Design review of the part shown in the three views and the two pictorial views. Dimensions are in mm from the part's minimum x, y and z. Give positions to 0.01 mm unless a question says otherwise; leave off trailing zeros. Order: outer loops, then holes, each group sorted by start corner. A loop starts at its lowest first (then second) coordinate and runs counter-clockwise, first axis right, second up.
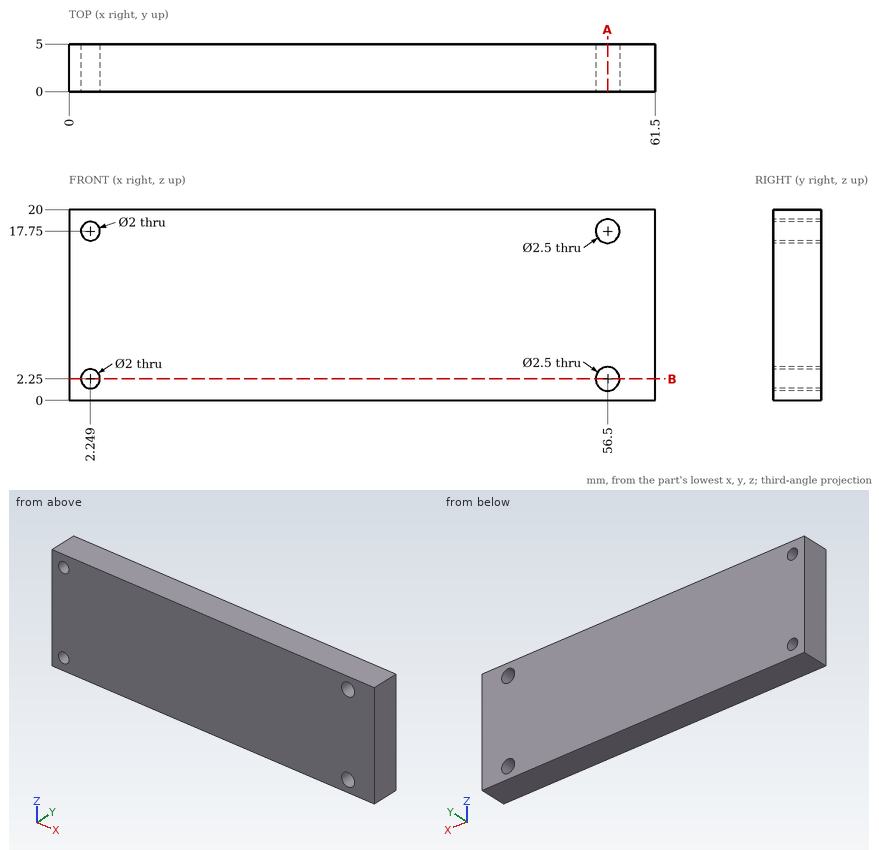
Item 1: Take a section at A-A (x = 56.5). Give the boundary of the cut face in (y, z), and give its area (3 significant figures).
Values found:
outline: (0, 0) - (5, 0) - (5, 1) - (0, 1) - close; (0, 3.5) - (5, 3.5) - (5, 16.5) - (0, 16.5) - close; (0, 19) - (5, 19) - (5, 20) - (0, 20) - close
area: 75.0 mm2
Item 2: Take a section at B-B (z = 2.25). Give the boundary of the cut face in (x, y).
Values found:
outline: (0, 0) - (1.25, 0) - (1.25, 5) - (0, 5) - close; (3.25, 0) - (55.25, 0) - (55.25, 5) - (3.25, 5) - close; (57.75, 0) - (61.5, 0) - (61.5, 5) - (57.75, 5) - close
Item 3: For line 1 (Z direction, x = 56.5, y = 1.25); line 2 (X direction, y = 3.15, z = 17.75); line 3 (X direction, y = 1.65, z = 18.5), list the stretches that pass through material, from the lowest coordinate up.
Values found:
line 1: z = 0 to 1, 3.5 to 16.5, 19 to 20
line 2: x = 0 to 1.25, 3.25 to 55.25, 57.75 to 61.5
line 3: x = 0 to 1.59, 2.91 to 55.5, 57.5 to 61.5
Item 4: Clearance check with flat-ended pins moving along their axes: pin 1 Ø3 at (x, z) = (56.5, 2.25) entering from +Y; pin 2 Ø1.8 at (x, z) = (2.249, 17.75) entering from -Y. State where each tip first meets the part, or that it passes through.
Values found:
pin 1: stops at y = 5
pin 2: passes through
